Autodesk Fusion 360 part; units mm, degrees
sketch "Sketch1" plane through (0, 0, 0) normal (0, 0, 1) x (1, 0, 0) in component "Mounting Plate1"
  line L0 (-50, 75) -> (50, 75)
  line L1 (50, 75) -> (50, -75)
  line L2 (50, -75) -> (-50, -75)
  line L3 (-50, -75) -> (-50, 75)
  line L4 (-50, 75) -> (50, -75) construction
  line L5 (50, 75) -> (-50, -75) construction
  circle A0 centre (-35, 60) radius 7.5
  circle A1 centre (35, 60) radius 7.5
  line L6 (0, 0) -> (21.7934, 0) construction
  circle A2 centre (-35, -60) radius 7.5
  circle A3 centre (35, -60) radius 7.5
  dimension "d1" = 100
  dimension "d2" = 150
  dimension "d3" = 15
  dimension "d4" = 15
  dimension "d5" = 15
  dimension "d6" = 15
extrude "Extrude1" add sketch "Sketch1" along normal blind 10 makes body 1 in component "Mounting Plate1"
fillet "Fillet1" radius 15 4 edges at (-50, 75, 5) (50, 75, 5) (50, -75, 5) (-50, -75, 5) on bodies 1 in component "Mounting Plate1"
ref_plane "WorkPlane1" through (0, -150, 0) normal (0, 1, 0) x (0, 0, 1) in component "Mounting Plate1"
sketch "Sketch2" plane through (0, -150, 0) normal (0, 1, 0) x (1, 0, 0) in component "Mounting Plate1"
  line L0 (-35, -10) -> (35, -10)
  line L1 (0, 0) -> (0, -125) construction
  line L2 (-50, -96.1325) -> (0, -182.735)
  line L3 (0, -182.735) -> (50, -96.1325)
  line L4 (50, -96.1325) -> (-50, -96.1325)
  point P0 (0, -125)
  dimension "d11" = 125
  dimension "d12" = 100
extrude "Extrude2" add sketch "Sketch2" against normal blind 10 separate body makes body 2 in component "Mounting Plate1"
fillet "Fillet2" radius 10 3 edges at (0, -155, 182.735) (50, -155, 96.1325) (-50, -155, 96.1325) on bodies 2 in component "Mounting Plate1"
sketch "Sketch3" plane through (0, 0, 0) normal (1, 0, 0) x (0, 0, -1) in component "Mounting Plate1"
  line L0 (-10, 75) -> (-10, -75)
  line L1 (-96.1325, -150) -> (-172.735, -150)
  arc A0 (-10, 27.5478) -> (-156.6245, -150) centre (77.7015, -194.1962) ccw
  arc A1 (-10, -23.3468) -> (-117.7051, -150) centre (74.486, -204.3157) ccw
extrude "Extrude3" add sketch "Sketch3" along normal mid plane 10 bodies 1 2 in component "Mounting Plate1"
component "Mounting Plate1" placed x (1, 0, 0) y (0, 1, 0) z (0, 0, 1) at (0, 0, 0)
equation "d2 = ( 6 * 25 ) * 1 mm"
Build history of the part. All positions in model axes, mm. A direction names the side the tool comes from. Give positions to 0.01 mm unless a question says otherwise; leave off trailing zeros. Loops run counter-clockwise (first coordinate to the right, second up) from the corner with the lowest first, then second, coordinate; pieces in that order, holes last.
Item 1: Slice it at C-C, the plane z = 139. List the corners of the cut face in (x, y).
Answers follow:
outline: (-25.25, -160) - (25.25, -160) - (25.25, -150) - (5, -150) - (5, -94.69) - (-5, -94.69) - (-5, -150) - (-25.25, -150) - close
Item 2: Pull direction Z, two halves, no side cores. Call faces 3 (the face through (-0.07, -75.85, 78.433)), 4 (the face through (0, 75, 5)), 5 (the face through (24.77, -154.93, 139.83)), 6 (the face through (-1, 1, 0)): released by +Z, released by -Z, zero draft, split by the parting line, or undercut.
Answers follow:
face 3: undercut
face 4: zero draft
face 5: released by +Z
face 6: released by -Z
Item 3: Slice it at A-A, the plane x = -20. List the corners of the cut face in (y, z).
Answers follow:
outline: (-160, 96.13) - (-150, 96.13) - (-150, 148.09) - (-160, 148.09) - close; (-75, 0) - (75, 0) - (75, 10) - (-75, 10) - close
Item 4: Drill centre lines: line 1 (Y direction, x = -35, z = 2); line 2 (Z direction, x = 21, y = -74.5); line 3 (Y direction, x = -36, z = 106). Where is each one in solid material? Low to high.
Answers follow:
line 1: y = -75 to -67.5, -52.5 to 52.5, 67.5 to 75
line 2: z = 0 to 10
line 3: y = -160 to -150
Item 5: Slice it at D-D, the plane y = -3. List the corners of the cut face in (x, z), and give its area (3 significant figures).
Answers follow:
outline: (-50, 0) - (50, 0) - (50, 10) - (5, 10) - (5, 64.8) - (-5, 64.8) - (-5, 10) - (-50, 10) - close
area: 1,550 mm2
Item 6: Flat gauge pins, fed straight in: pin 1 (5 mm diameter, centred on x = -16.5, y = -58.5, fed in from +Z); pin 2 (3 mm diameter, centred on x = -14, z = 4, fed in from -Y); pin 3 (10 mm diameter, centred on x = 32.5, y = -53, fed in from -Z); pin 4 (8 mm diameter, centred on x = 2, y = -45.5, fed in from +Z). Where does each tip first touch, or does it go through?
Answers follow:
pin 1: stops at z = 10
pin 2: stops at y = -75
pin 3: stops at z = 0
pin 4: stops at z = 111.84
Item 7: Slice it at B-B, the plane y = -63. List the corners of the cut face in (x, z), and give its area (3 significant figures).
Answers follow:
outline: (-49.7, 0) - (-41.87, 0) - (-41.87, 10) - (-49.7, 10) - close; (-28.13, 0) - (28.13, 0) - (28.13, 10) - (-28.13, 10) - close; (-5, 66.64) - (5, 66.64) - (5, 121.42) - (-5, 121.42) - close; (41.87, 0) - (49.7, 0) - (49.7, 10) - (41.87, 10) - close
area: 1,270 mm2
Item 8: Which spindle directions (+Z, -Z, +X, -X, +Y, -Y) get a long thin tool onto all of the face, cutting with end or side? Do faces 1 (the face through (-5, -61, 84)), 2 (the face through (0.147, -155.07, 172.734)). Say none if no direction does.
Answers follow:
face 1: +Z, -X, +Y
face 2: +Z, +Y, -Y
